Here's the drawing with two shaded views (mm, measured from the low corner). I have some questions. A direction names the side the tool comes from. Coordinates: 2 decimals unless noted, no trailing zeros. Loops run counter-clockwise (first coordinate to the right, second up) from the corner with the lowest first, then second, coordinate; pieces in that order, holes last. Notation, with made-up numbers: (38.25, 82) - (69.25, 82) arc R22 cw to (69.25, 120) - close; hole circle Ø9 at (54.5, 50.5). An arc over 180 degrees is marked (long way). Use a Markdown table: item, result.
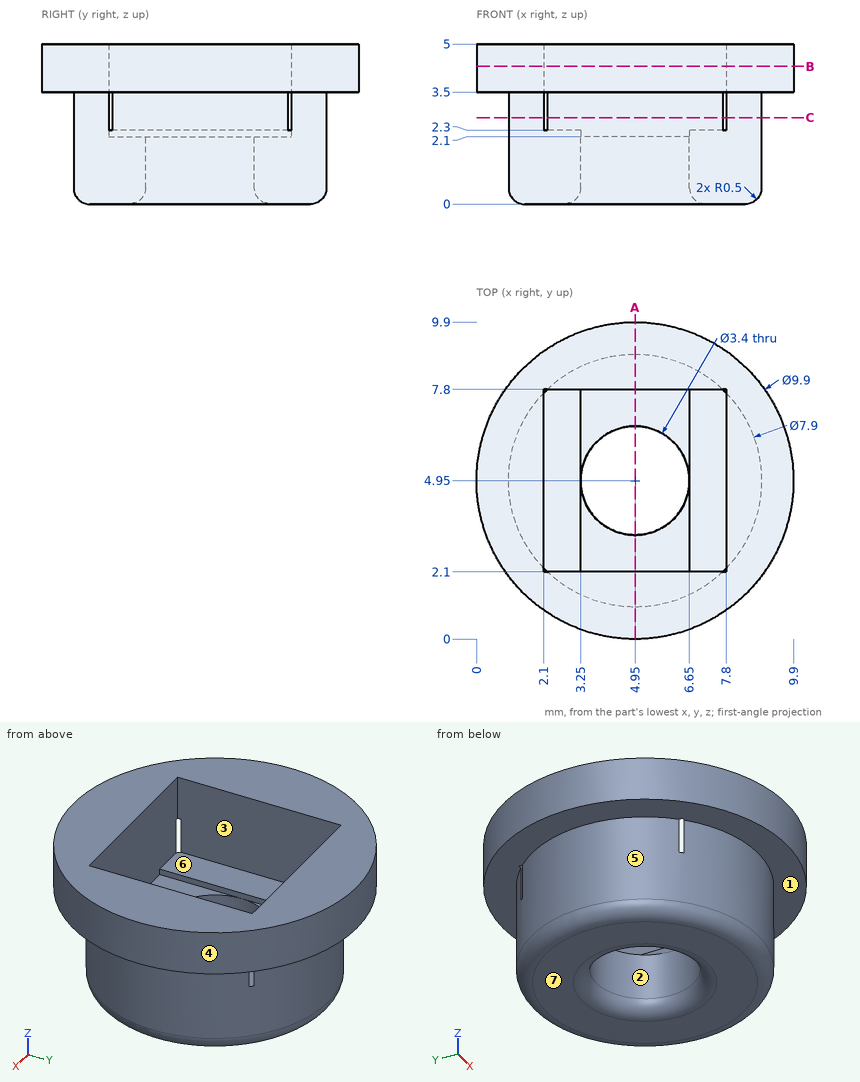
Q1. Which directions (+Z, -Z, +X, -X, +Y, -Y) give clear straight access to the entire face, cutting with the end or side of a thin tool? Please do the marked faces 5, 6 and 7.
Check values:
| item | result |
|---|---|
| face 5 | -Z |
| face 6 | +Z |
| face 7 | -Z, +X, -X, +Y, -Y |
Q2. Please list where these lines run through material, in increasing order: L1, parallel to Y at x = 5, z = 3.8; L2, parallel to Y at x = 4.95, z = 1.15; L3, parallel to Z at x = 9, y = 5.75. Write a range as from..to.
Check values:
| item | result |
|---|---|
| L1 | 0..2.1, 7.8..9.9 |
| L2 | 1..3.25, 6.65..8.9 |
| L3 | 3.5..5 |
Q3. Will these pins go through, and if not, where does the flat tip stop? P1, Ø0.9, axis at x = 5.5, z = 4, coming from the +Y side; P2, Ø1.4, axis at x = 5.5, y = 3.5, coming from the +Z side; P3, Ø3, axis at x = 6, y = 4.5, coming from the +Z side.
Check values:
| item | result |
|---|---|
| P1 | y = 9.9 |
| P2 | z = 2.1 |
| P3 | z = 2.3 |
Q4. I want a section at B-B, the plane z = 4.3. Write out the boundary of the cut face in (x, y).
Check values:
| item | result |
|---|---|
| outline | circle Ø9.9 at (4.95, 4.95); hole (2.1, 2.1) - (7.8, 2.1) - (7.8, 7.8) - (2.1, 7.8) - close |
Q5. I want a section at A-A, the plane x = 4.95. Write out the boundary of the cut face in (y, z), then the cut area to 3 significant figures.
Check values:
| item | result |
|---|---|
| outline | (0, 3.5) - (1, 3.5) - (1, 0.5) arc R0.5 ccw to (1.5, 0) - (2.75, 0) arc R0.5 ccw to (3.25, 0.5) - (3.25, 2.1) - (2.1, 2.1) - (2.1, 5) - (0, 5) - close; (6.65, 0.5) arc R0.5 ccw to (7.15, 0) - (8.4, 0) arc R0.5 ccw to (8.9, 0.5) - (8.9, 3.5) - (9.9, 3.5) - (9.9, 5) - (7.8, 5) - (7.8, 2.1) - (6.65, 2.1) - close |
| area | 18.6 mm^2 |
Q6. I want a section at C-C, the plane z = 2.7. Write out the boundary of the cut face in (x, y).
Check values:
| item | result |
|---|---|
| outline | (2.1, 2.22) - (2.1, 7.68) arc R3.95 ccw to start; (2.22, 2.1) arc R3.95 ccw to (7.68, 2.1) - close; (2.22, 7.8) - (7.68, 7.8) arc R3.95 ccw to start; (7.8, 2.22) arc R3.95 ccw to (7.8, 7.68) - close |
Q7. If we mould it in two halves opening along Y, with no side actions, what happens to the marked faces 1, 2, 3 and 4? For each: pulls with the +Y half, pulls with the -Y half, needs draft (parallel to the pull), parting line crosses it, or undercut.
Check values:
| item | result |
|---|---|
| face 1 | needs draft |
| face 2 | undercut |
| face 3 | undercut |
| face 4 | parting line crosses it |
